Source: CAD feature listing. Evaluate the final solid. Frame: model axes, mm. A direction names the side the tool comes from. Give positions to 0.01 mm unless a question says otherwise; leave off trailing zeros. Write each loop counter-clockwise with the first axis right and the second up, starting at its lowest first coordinate (ties: lowest second). Pieces come first, ordered by that corner, then holes. Notation, with made-up numbers: (-2, 83.25) -> (20, 83.25) arc R25 cw to (20, 97.25) -> close; hole circle Ø2 at (18, -23). An arc over 180 degrees is marked (long way). Answer as a JSON object with one key per item and string values. Group by question number.
Item 1: Section query C-C on y = 3.81. Return the cut outline in (x, z).
Item 2: Pull-direction query (Z, two-part tool) for faces 1 (the face through (-10.224, -18.649, 7.534)), 2 (the face through (150.089, 0, 27)), 3 (the face through (138, 0, 44.45)), 4 (the face through (-8.87, -18.44, -6.8)); classes: pulls with the +Z half, pulls with the -Z half, needs draft (parallel to the pull), parting line crosses it, or undercut.
Item 3: Section query A-A on y = -5. Return the cut outline in (x, z), plus the area to 3 significant figures.
Item 4: First-contact query: pin 1 Ø16.5 at (x, y) = (165, 3.81) entering from +Z; pin 2 Ø1.5 at (x, z) = (112, -3.5) entering from -Y; pin 3 Ø18 at (x, z) = (0, 0) entering from +Y; pin 4 Ø15.5 at (x, y) = (86, 9) entering from +Z. Flat tips, straight axial feed; report the tip coordinate or a pass-through.
Item 5: Section query B-B on x = 58.5. Return the cut outline in (y, z), plus the area to 3 significant figures.
Item 6: Ray query, probe 1 along Z at (x, y) = (0, -14); probe 2 along X at (y, z) = (22, 0); probe 3 along X at (y, z) = (-20.5, 8.5). Return the intervals inside material, ascending. Write a range as from..to.
Item 7: Section query D-D on z = 30.5. Return the cut outline in (x, y).
Item 8: Access query for faces 5 (the face through (128.595, -0.366, 23.257)), 6 (the face through (117.246, -13, -4)), 7 (the face through (101, 0, -4)), 8 (the face through (176, 0, 9.652)). Directions: +Z, -Z, +X, -X, +Y, -Y. A direction counts if a zero-diameter tool reaches every point of the face in a straight line with its end or side. Return the directions, or none.
from build123d import *

# Parameters (mm, degrees)
F0_R     = 11.176
F1_DEPTH = 26.162
F2_DEPTH = 26.163
F3_R     = 12.739133
F4_DEPTH = 10.922
F5_R     = 6.35
F6_DEPTH = 22.353


with BuildPart() as f1:
    # F0 (on Front) → F1 (new body, symmetric)
    with BuildSketch(Plane.XZ):
        with BuildLine():
            Line((85.852, 4.49157), (11.879217, 4.49157))
            ThreePointArc((11.879217, 4.49157), (-10.448276, 7.219663), (0, -12.7))
            Line((0, -12.7), (91.8464, -12.7))
            Line((91.8464, -12.7), (85.852, 4.49157))
        make_face()
        Circle(F0_R, mode=Mode.SUBTRACT)
        Polygon((117.2464, 4.49157), (85.852, 4.49157), (91.8464, -12.7), (117.2464, -12.7), (117.2464, 1.780633), align=None)
        Polygon((117.2464, 1.780633), (117.2464, -12.7), (203.864659, -12.7), (203.859816, 1.780633), align=None)
        with BuildLine():
            ThreePointArc((131.0386, 44.45), (128.496139, 22.968067), (117.2464, 4.49157))
            Line((117.2464, 4.49157), (117.2464, 1.780633))
            Line((117.2464, 1.780633), (203.859816, 1.780633))
            ThreePointArc((203.859816, 1.780633), (201.552644, 7.34669), (195.985816, 9.652))
            Line((195.985816, 9.652), (155.1686, 9.652))
            ThreePointArc((155.1686, 9.652), (151.576498, 11.139898), (150.0886, 14.732))
            Line((150.0886, 14.732), (150.0886, 39.37))
            ThreePointArc((150.0886, 39.37), (148.600702, 42.962102), (145.0086, 44.45))
            Line((145.0086, 44.45), (131.0386, 44.45))
        make_face()
    extrude(amount=F1_DEPTH, both=True)

    # F0 (on Front) → F2 (cut, through all)
    with BuildSketch(Plane.XZ):
        Polygon((117.2464, 4.49157), (85.852, 4.49157), (91.8464, -12.7), (117.2464, -12.7), (117.2464, 1.780633), align=None)
    extrude(amount=F2_DEPTH, mode=Mode.SUBTRACT)

    # F3 (on Front) → F4 (cut, symmetric)
    with BuildSketch(Plane.XZ):
        Circle(F3_R)
    extrude(amount=F4_DEPTH, both=True, mode=Mode.SUBTRACT)

    # F5 (on face) → F6 (cut, through all)
    with BuildSketch(Plane.XY.offset(9.652)):
        with Locations((164.997816, 3.81)):
            Circle(F5_R)
    extrude(amount=-F6_DEPTH, mode=Mode.SUBTRACT)


solid = f1.part
Worked answers:
{
 "1": {"outline": "(1, -12.7) -> (158.65, -12.7) -> (158.65, 9.65) -> (155.17, 9.65) arc R5.08 cw to (150.09, 14.73) -> (150.09, 39.37) arc R5.08 ccw to (145.01, 44.45) -> (131.04, 44.45) arc R50.8 cw to (117.25, 4.49) -> (11.92, 4.49) arc R12.74 cw to start; (171.35, -12.7) -> (203.86, -12.7) -> (203.86, 1.78) arc R7.87 ccw to (195.99, 9.65) -> (171.35, 9.65) -> close"},
 "2": {"face 1": "parting line crosses it", "face 2": "needs draft", "face 3": "pulls with the +Z half", "face 4": "undercut"},
 "3": {"outline": "(1, -12.7) -> (91.85, -12.7) -> (85.85, 4.49) -> (11.92, 4.49) arc R12.74 cw to start; (117.25, -12.7) -> (203.86, -12.7) -> (203.86, 1.78) arc R7.87 ccw to (195.99, 9.65) -> (155.17, 9.65) arc R5.08 cw to (150.09, 14.73) -> (150.09, 39.37) arc R5.08 ccw to (145.01, 44.45) -> (131.04, 44.45) arc R50.8 cw to (117.25, 4.49) -> close", "area": "4,000 mm^2"},
 "4": {"pin 1": "z = 9.65", "pin 2": "y = 0", "pin 3": "through", "pin 4": "z = 4.49"},
 "5": {"outline": "(-26.16, -12.7) -> (26.16, -12.7) -> (26.16, 4.49) -> (-26.16, 4.49) -> close", "area": "900 mm^2"},
 "6": {"probe 1": "-12.7..-11.18, 11.18..12.7", "probe 2": "-12.7..-11.18, 11.18..203.86", "probe 3": "-9.44..-7.26, 7.26..9.44, 120.69..200.09"},
 "7": {"outline": "(130.46, -26.16) -> (150.09, -26.16) -> (150.09, 26.16) -> (130.46, 26.16) -> close"},
 "8": {"face 5": "+Y, -Y", "face 6": "+Z, -Z, -Y", "face 7": "+Z, -Y", "face 8": "+Z, +X, +Y, -Y"}
}
